from build123d import *

# Parameters (mm, degrees)
F3_DEPTH        = 9
F3_COPIES_COUNT = 16


# Not quite as in the source:
# - a pattern or mirror of a feature is missing from the dataset's text; its kind, count and spacing are read off the source's solid


with BuildPart() as f1:
    # F0 (on Front) → F1 (revolve)
    with BuildSketch(Plane.XZ):
        Polygon((20, 12), (20, 0), (29.0510931471, 0), (29.0510931471, 3), (21.25, 3), (21.25, 12), align=None)
    revolve(axis=Axis((0, 0, 7.2627740937), (0, 0, 1)))

    # F2 (on face) → F3 (join, through all)
    with BuildSketch(Plane.XY.offset(3)):
        with BuildLine():
            ThreePointArc((-0.9737363442, 21.2276785714), (0, 21.25), (0.9737363442, 21.2276785714))
            ThreePointArc((0.9737363442, 21.2276785714), (0, 22), (-0.9737363442, 21.2276785714))
        make_face()
    f3 = extrude(amount=F3_DEPTH)

    # F3_copies: F3 ×16 about axis
    f3_copies_axis = Axis((0, 0, 0), (0, 0, 1))
    for i in range(1, F3_COPIES_COUNT):
        add(f3.rotate(f3_copies_axis, i * 360 / F3_COPIES_COUNT))


solid = f1.part
Can you work these out from the model? Positions are in its coordinate system, mm. A direction names the side the tool comes from. Round coordinates to 2 decimals unless told otherwise and drop trailing zeros. Write each loop counter-clockwise with the first axis right and the second up, starting at its lowest first coordinate (ties: lowest second). Pieces come first, ordered by that corner, then holes. Notation, with made-up numbers: (-6.5, 26) - (51.5, 26) arc R20 cw to (51.5, 52) - close; hole circle Ø2 at (73, 61). An arc over 180 degrees is marked (long way). Write each question's results on one line, items separated by ' | '. Start each with the question number.
1) Which directions (+Z, -Z, +X, -X, +Y, -Y) give clear straight access to the entire face, cutting with the end or side of a thin tool? Please do faces 4 (the flat face through (-13, 17, 3)), 5 (the cylindrical face through (-4.1, 20.85, 7.56)), 6 (the cylindrical face through (-20.833, 4.19, 7.563)), 7 (the cylindrical face through (20.833, -4.19, 7.563)).
2) Please list where these lines run through material, in increasing order: line 1 (Y direction, x = 0, z = 6.5); line 2 (Z direction, x = 21, y = 9); line 3 (Y direction, x = -3.5, z = 6.75).
3) For pin 1 Ø12 at (x, y) = (2.5, -12) entering from -Z; pin 2 Ø4 at (y, z) = (-10, 8) entering from +X; pin 3 Ø2 at (y, z) = (-18, 6.5) entering from -X; pin 4 Ø2 at (y, z) = (22.5, 1.5) entering from -X, each with a flat end and sliding along its axis, tell me the tip position at first contact or that it passes through.
4) We'd pull the mould along Y, two halves only. Please class faces 1 (the cylindrical face through (4.19, 20.833, 7.563)), 2 (the cylindrical face through (-20.318, 8.436, 7.437)), 3 (the cylindrical face through (22, 0, 7)): released by +Y, released by -Y, zero draft, split by the parting line, or undercut.
5) Suppose I cut it at A-A (y = 0). List the corners of the cut face in (x, z) for me, and give its area (3 significant figures).
6) Suppose I cut it at D-D (y = 23.5). List the corners of the cut face in (x, z) for me, and give its area (3 significant figures).
Here are the results:
1) face 4: +Z | face 5: +Z, +Y | face 6: +Z, -X | face 7: +Z, +X
2) line 1: y = -22 to -20, 20 to 22 | line 2: z = 0 to 3 | line 3: y = -20.96 to -19.69, 19.69 to 20.96
3) pin 1: passes through | pin 2: stops at x = 20.4 | pin 3: stops at x = -12.75 | pin 4: stops at x = -19.54
4) face 1: released by +Y | face 2: undercut | face 3: split by the parting line
5) outline: (-29.05, 0) - (-20, 0) - (-20, 12) - (-22, 12) - (-22, 3) - (-29.05, 3) - close; (20, 0) - (29.05, 0) - (29.05, 3) - (22, 3) - (22, 12) - (20, 12) - close | area: 90.3 mm2
6) outline: (-17.08, 0) - (17.08, 0) - (17.08, 3) - (-17.08, 3) - close | area: 102 mm2
